Read the model definition and answer for the solid it produces. Units are mm, in the model's axes. Coordinates: 2 decimals unless noted, no trailing zeros. Write each loop counter-clockwise with the first axis right and the second up, starting at its lowest first coordinate (ties: lowest second). Pieces come first, ordered by that corner, then holes. Notation, with made-up numbers: (14, 25) -> (53, 25) arc R10 cw to (53, 41) -> close; hole circle Ø8 at (44.5, 80). An arc over 180 degrees is marked (long way). Return JSON: item names as keys, results as strings.
from build123d import *

# Parameters (mm, degrees)
BOSS_EXTRUDE1_DEPTH  = 138
MIRROR3_COPY_1_DEPTH = 138
MIRROR3_COPY_2_DEPTH = 138


with BuildPart() as part:
    # Sketch1 → Boss-Extrude1 (new body)
    with BuildSketch(Plane.XY):
        with BuildLine():
            Line((3.4, 0), (5.5, 0))
            Line((5.5, 0), (5.5, 4))
            Line((5.5, 4), (11.69, 10.19))
            Line((11.69, 10.19), (18.2, 10.19))
            Line((18.2, 10.19), (18.2, 5.265595036))
            Line((18.2, 5.265595036), (15.5, 5.265595036))
            Line((15.5, 5.265595036), (15.5, 2.965595036))
            Line((15.5, 2.965595036), (19, 2.965595036))
            Line((19, 2.965595036), (19, 3.965595036))
            Line((19, 3.965595036), (20, 3.965595036))
            Line((20, 3.965595036), (20, 15.5))
            ThreePointArc((20, 15.5), (18.681980515, 18.681980515), (15.5, 20))
            Line((15.5, 20), (6.385304712, 20))
            Line((6.385304712, 20), (6.385304712, 19))
            Line((6.385304712, 19), (5.385304712, 19))
            Line((5.385304712, 19), (5.385304712, 15.5))
            Line((5.385304712, 15.5), (7.685304712, 15.5))
            Line((7.685304712, 15.5), (7.685304712, 18.2))
            Line((7.685304712, 18.2), (10.19, 18.2))
            Line((10.19, 18.2), (10.19, 11.69))
            Line((10.19, 11.69), (4, 5.5))
            Line((4, 5.5), (0, 5.5))
            Line((0, 5.5), (0, 3.4))
            ThreePointArc((0, 3.4), (2.404163056, 2.404163056), (3.4, 0))
        make_face()
        with BuildLine():
            Line((18.5, 11.69), (18.5, 15.5))
            ThreePointArc((18.5, 15.5), (17.621320344, 17.621320344), (15.5, 18.5))
            Line((15.5, 18.5), (11.69, 18.5))
            Line((11.69, 18.5), (11.69, 11.69))
            Line((11.69, 11.69), (18.5, 11.69))
        make_face(mode=Mode.SUBTRACT)
    boss_extrude1 = extrude(amount=BOSS_EXTRUDE1_DEPTH)

    # Mirror1: Boss-Extrude1 across plane
    add(boss_extrude1.mirror(Plane.ZX))

    # Mirror2: Boss-Extrude1 across plane
    add(boss_extrude1.mirror(Plane(origin=(0, 0, 0), x_dir=(0, 0, 1), z_dir=(1, 0, 0))))

    # Mirror3 copy 1 sketch → Mirror3 copy 1 (add)
    with BuildSketch(Plane(origin=(0, 0, 0), x_dir=(-1, 0, 0), z_dir=(0, 0, 1))):
        with BuildLine():
            Line((3.4, 0), (5.5, 0))
            Line((5.5, 0), (5.5, 4))
            Line((5.5, 4), (11.69, 10.19))
            Line((11.69, 10.19), (18.2, 10.19))
            Line((18.2, 10.19), (18.2, 5.265595036))
            Line((18.2, 5.265595036), (15.5, 5.265595036))
            Line((15.5, 5.265595036), (15.5, 2.965595036))
            Line((15.5, 2.965595036), (19, 2.965595036))
            Line((19, 2.965595036), (19, 3.965595036))
            Line((19, 3.965595036), (20, 3.965595036))
            Line((20, 3.965595036), (20, 15.5))
            ThreePointArc((20, 15.5), (18.681980515, 18.681980515), (15.5, 20))
            Line((15.5, 20), (6.385304712, 20))
            Line((6.385304712, 20), (6.385304712, 19))
            Line((6.385304712, 19), (5.385304712, 19))
            Line((5.385304712, 19), (5.385304712, 15.5))
            Line((5.385304712, 15.5), (7.685304712, 15.5))
            Line((7.685304712, 15.5), (7.685304712, 18.2))
            Line((7.685304712, 18.2), (10.19, 18.2))
            Line((10.19, 18.2), (10.19, 11.69))
            Line((10.19, 11.69), (4, 5.5))
            Line((4, 5.5), (0, 5.5))
            Line((0, 5.5), (0, 3.4))
            ThreePointArc((0, 3.4), (2.404163056, 2.404163056), (3.4, 0))
        make_face()
        with BuildLine():
            Line((18.5, 11.69), (18.5, 15.5))
            ThreePointArc((18.5, 15.5), (17.621320344, 17.621320344), (15.5, 18.5))
            Line((15.5, 18.5), (11.69, 18.5))
            Line((11.69, 18.5), (11.69, 11.69))
            Line((11.69, 11.69), (18.5, 11.69))
        make_face(mode=Mode.SUBTRACT)
    extrude(amount=MIRROR3_COPY_1_DEPTH)

    # Mirror3 copy 2 sketch → Mirror3 copy 2 (add)
    with BuildSketch(Plane.XY):
        with BuildLine():
            Line((3.4, 0), (5.5, 0))
            Line((5.5, 0), (5.5, -4))
            Line((5.5, -4), (11.69, -10.19))
            Line((11.69, -10.19), (18.2, -10.19))
            Line((18.2, -10.19), (18.2, -5.265595036))
            Line((18.2, -5.265595036), (15.5, -5.265595036))
            Line((15.5, -5.265595036), (15.5, -2.965595036))
            Line((15.5, -2.965595036), (19, -2.965595036))
            Line((19, -2.965595036), (19, -3.965595036))
            Line((19, -3.965595036), (20, -3.965595036))
            Line((20, -3.965595036), (20, -15.5))
            ThreePointArc((20, -15.5), (18.681980515, -18.681980515), (15.5, -20))
            Line((15.5, -20), (6.385304712, -20))
            Line((6.385304712, -20), (6.385304712, -19))
            Line((6.385304712, -19), (5.385304712, -19))
            Line((5.385304712, -19), (5.385304712, -15.5))
            Line((5.385304712, -15.5), (7.685304712, -15.5))
            Line((7.685304712, -15.5), (7.685304712, -18.2))
            Line((7.685304712, -18.2), (10.19, -18.2))
            Line((10.19, -18.2), (10.19, -11.69))
            Line((10.19, -11.69), (4, -5.5))
            Line((4, -5.5), (0, -5.5))
            Line((0, -5.5), (0, -3.4))
            ThreePointArc((0, -3.4), (2.404163056, -2.404163056), (3.4, 0))
        make_face()
        with BuildLine():
            Line((18.5, -11.69), (18.5, -15.5))
            ThreePointArc((18.5, -15.5), (17.621320344, -17.621320344), (15.5, -18.5))
            Line((15.5, -18.5), (11.69, -18.5))
            Line((11.69, -18.5), (11.69, -11.69))
            Line((11.69, -11.69), (18.5, -11.69))
        make_face(mode=Mode.SUBTRACT)
    extrude(amount=MIRROR3_COPY_2_DEPTH)


solid = part.part
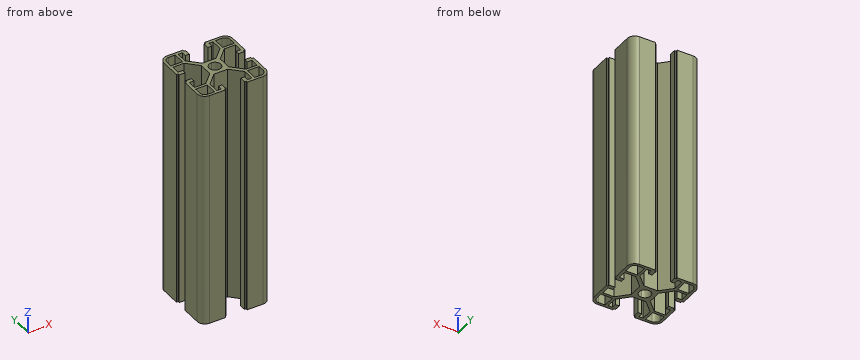
1. The part is cut by section C-C (z = 88). Count the separate pieces of the cut face and the enclosed holes in it, then the cut area to 3 significant figures.
Taken from the geometry:
{"separate pieces": "1", "enclosed holes": "5", "area": "468 mm2"}
2. A flat-ended cylindrical pin translates along its axis: pin 1 Ø2 at (x, z) = (-17.5, 37) entering from +Y. Find the tip coordinate at first contact, or state that the pin passes through.
Taken from the geometry:
{"pin 1": "stops at y = 19.89"}
3. Consider L1, parallel to X at y = 3.5, z = 84; L2, parallel to Y at x = -12, z = 39. Determine where each line is inside the solid, lowest interval first.
Taken from the geometry:
{"L1": "x = -19 to -15.5, -5.5 to 5.5, 15.5 to 19", "L2": "y = -20 to -18.5, -11.69 to -10.19, 10.19 to 11.69, 18.5 to 20"}
4. The part is cut by section A-A (x = 13). Determine the outline of the cut face in (y, z), then the cut area to 3 significant figures.
Taken from the geometry:
{"outline": "(-20, 0) -> (-18.5, 0) -> (-18.5, 138) -> (-20, 138) -> close; (-11.69, 0) -> (-10.19, 0) -> (-10.19, 138) -> (-11.69, 138) -> close; (10.19, 0) -> (11.69, 0) -> (11.69, 138) -> (10.19, 138) -> close; (18.5, 0) -> (20, 0) -> (20, 138) -> (18.5, 138) -> close", "area": "828 mm2"}
5. The part is cut by section B-B (y = 7.5). Determine the outline of the cut face in (x, z), then the cut area to 3 significant figures.
Taken from the geometry:
{"outline": "(-20, 0) -> (-18.2, 0) -> (-18.2, 138) -> (-20, 138) -> close; (-9, 0) -> (-6, 0) -> (-6, 138) -> (-9, 138) -> close; (6, 0) -> (9, 0) -> (9, 138) -> (6, 138) -> close; (18.2, 0) -> (20, 0) -> (20, 138) -> (18.2, 138) -> close", "area": "1,320 mm2"}
